Can you work these out from the drawing? Everything is in mm from the part's minimum corner. Round coordinates to 2 decimals unless told otherwise and drop trailing zeros. Loops run counter-clockwise (first coordinate to the right, second up) from the corner with the lowest first, then second, coordinate; pieces in that order, holes last. Notation, with made-up numbers: (12, 14) - (50, 14) arc R16 ccw to (50, 34) - close; hole circle Ø2 at (62, -22). An arc over 180 degrees is marked (long way). Return JSON: item names as keys, results as strings. Group by question number.
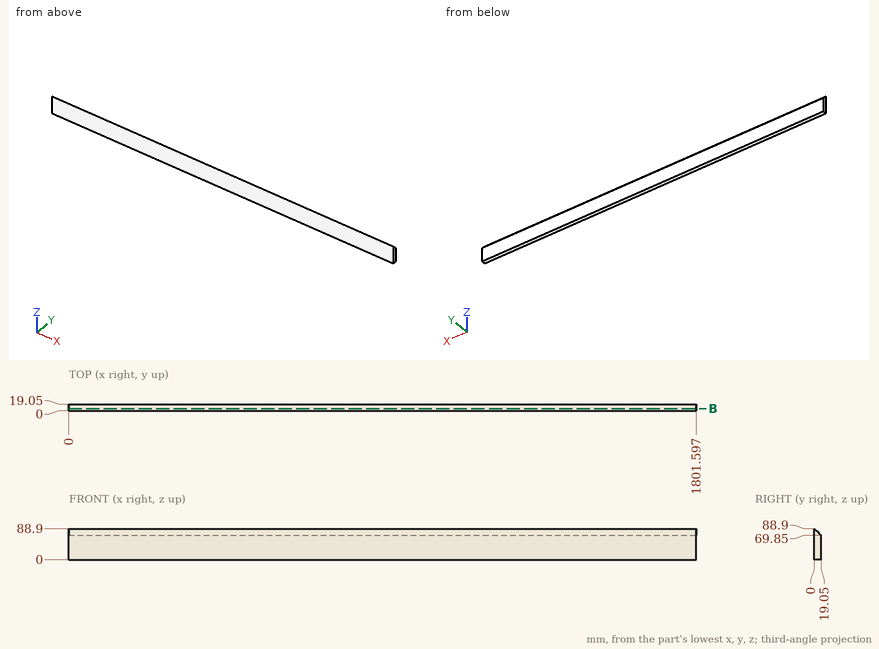
Q1. Will these pins go through, and if not, where does the flat tip stop? pin 1 Ø1 at (x, y) = (539.5, 16.5) entering from +Z; pin 2 Ø2 at (x, y) = (1322, 14) entering from +Z.
Q2. Imagine slicing it at B-B, the plane y = 6. List the corners of the cut face in (x, z) for me, and give its area (3 significant figures).
Q3. Please list where these lines run through material, in increasing order: line 1 (Z direction, x = 850, y = 6.5); line 2 (Z direction, x = 1142, y = 18.75); line 3 (Y direction, x = 1679, z = 70.5).
Output values:
{
 "1": {"pin 1": "stops at z = 72.9", "pin 2": "stops at z = 75.9"},
 "2": {"outline": "(0, 0) - (1801.6, 0) - (1801.6, 82.9) - (0, 82.9) - close", "area": "149,000 mm^2"},
 "3": {"line 1": "z = 0 to 82.4", "line 2": "z = 0 to 70.15", "line 3": "y = 0 to 18.4"}
}
